Answer from the drawing. Dimensions are ordinates in mm from the lowest x, y and z of the part. Round coordinates to 2 decimals unless told otherwise and drop trailing zeros. Order: outer loops, then holes, each group sorted by start corner. A loop starts at its lowest first (then second) coordinate and runs counter-clockwise, first axis right, second up.
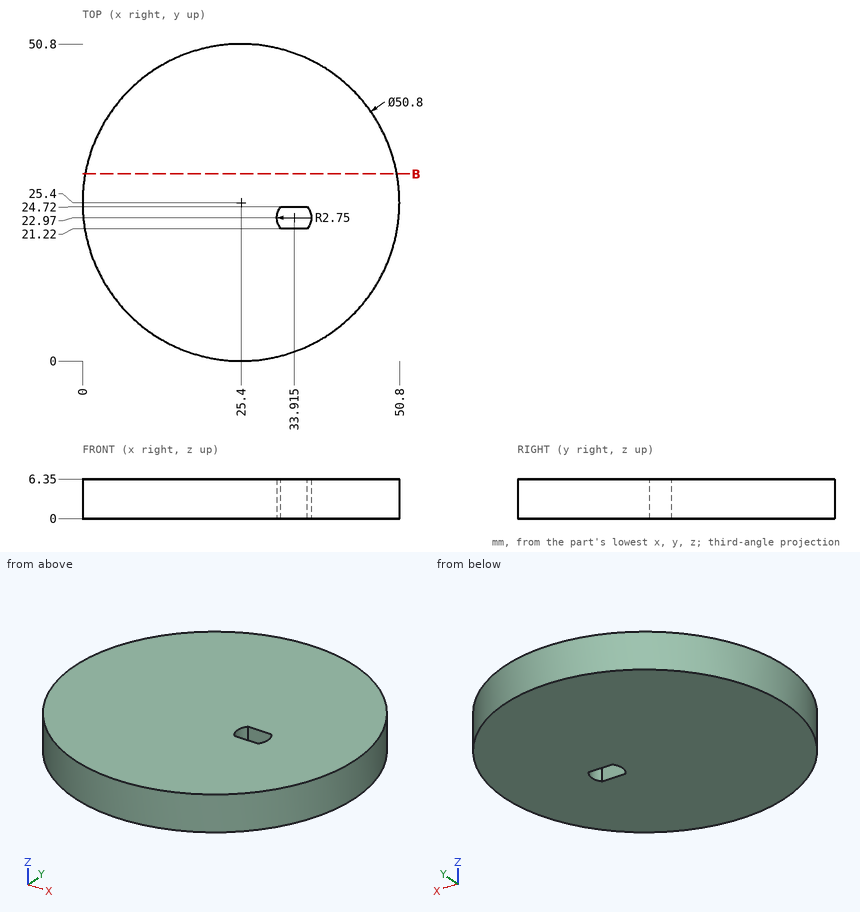
Q1. Straight lines are drawn through the part: probe 1 along Y at (x, z) = (25.5, 0.5); probe 2 along X at (y, z) = (23.5, 1.5) (1 decimal); probe 3 along Y at (x, z) = (34.5, 1.75) (1 decimal). For each, find the intervals that lie inside material, in ascending order.
Outcome:
probe 1: y = 0 to 50.8
probe 2: x = 0.1 to 31.2, 36.6 to 50.7
probe 3: y = 1.7 to 21.2, 24.7 to 49.1
Q2. Flat-ended cylindrical pins translate along their axes: pin 1 (1 mm diameter, centred on y = 17, z = 5.5, fed in from +X); pin 2 (3 mm diameter, centred on y = 11.5, z = 1.5, fed in from +X); pin 3 (2 mm diameter, centred on x = 33.5, z = 4, fed in from -Y). Find the tip coordinate at first contact, or state that the pin passes through.
Outcome:
pin 1: stops at x = 49.54
pin 2: stops at x = 47.57
pin 3: stops at y = 1.01
Q3. A cutting plane is placed at B-B, the plane y = 30. Give the vertices of the cut face in (x, z).
Outcome:
outline: (0.42, 0) - (50.38, 0) - (50.38, 6.35) - (0.42, 6.35) - close
